The listing builds one solid part. Answer for the finished solid, in the listing's coordinates (mm). Face numbers are marked on the shaded views. A direction names the side the tool comes from. Coordinates: 2 decimals unless noted, no trailing zeros. Loops run counter-clockwise (first coordinate to the right, second up) from the corner with the lowest first, then second, coordinate; pieces in that order, holes last. Notation, with made-up numbers: (74, 51) -> (83, 51) arc R22 cw to (83, 65) -> close; hole circle Ø2 at (-38.75, -17). An arc over 180 degrees is marked (long way). Answer in a Markdown table with one row per item.
```python
from build123d import *

# Parameters (mm, degrees)
SKETCH1_R                                         = 40
SKETCH1_R_2                                       = 26
BOSS_EXTRUDE1_DEPTH                               = 82
BOSS_EXTRUDE2_DEPTH                               = 20
SKETCH4_R                                         = 26
CUT_EXTRUDE1_DEPTH                                = 22
CBORE_FOR_M10_HEX_HEAD_BOLT2_D                    = 13
CBORE_FOR_M10_HEX_HEAD_BOLT2_CBORE_D              = 22
CBORE_FOR_M10_HEX_HEAD_BOLT2_CBORE_DEPTH          = 8
FILLET1_R                                         = 8
CSK_FOR_M10_FLAT_HEAD_MACHINE_SCREW12_D           = 10
CSK_FOR_M10_FLAT_HEAD_MACHINE_SCREW12_DEPTH       = 30
CSK_FOR_M10_FLAT_HEAD_MACHINE_SCREW12_CSINK_D     = 22
CSK_FOR_M10_FLAT_HEAD_MACHINE_SCREW12_CSINK_ANGLE = 50
CSK_FOR_M10_FLAT_HEAD_MACHINE_SCREW12_TIP         = 3.004303095
SKETCH22_R                                        = 30
CUT_EXTRUDE2_DEPTH                                = 6


with BuildPart() as part:
    # Sketch1 → Boss-Extrude1 (new body)
    with BuildSketch(Plane(origin=(0, 0, 0), x_dir=(0, 1, 0), z_dir=(0, 0, 1))):
        with Locations(Location((0, 0, 0), (0, 0, 270))):
            Circle(SKETCH1_R)
        with Locations(Location((0, 0, 0), (0, 0, 270))):
            Circle(SKETCH1_R_2, mode=Mode.SUBTRACT)
    extrude(amount=BOSS_EXTRUDE1_DEPTH)

    # Sketch2 → Boss-Extrude2 (add)
    with BuildSketch(Plane(origin=(0, 0, 0), x_dir=(0, 1, 0), z_dir=(0, 0, 1))):
        with BuildLine():
            Line((-73.617309286, 3.070026527), (-11.117309286, 72.070026527))
            ThreePointArc((-11.117309286, 72.070026527), (0, 77), (11.117309286, 72.070026527))
            Line((11.117309286, 72.070026527), (73.617309286, 3.070026527))
            ThreePointArc((73.617309286, 3.070026527), (76.212228081, -13.080690837), (62.5, -22))
            Line((62.5, -22), (33.406586177, -22))
            ThreePointArc((33.406586177, -22), (0, -40), (-33.406586177, -22))
            Line((-33.406586177, -22), (-62.5, -22))
            ThreePointArc((-62.5, -22), (-76.212228081, -13.080690837), (-73.617309286, 3.070026527))
        make_face()
    extrude(amount=BOSS_EXTRUDE2_DEPTH)

    # Sketch4 → Cut-Extrude1 (cut)
    with BuildSketch(Plane.XY.offset(20)):
        Circle(SKETCH4_R)
    extrude(amount=-CUT_EXTRUDE1_DEPTH, mode=Mode.SUBTRACT)

    # CBORE for M10 Hex Head Bolt2 (through all)
    with Locations(Plane(origin=(-62, 0, 20), x_dir=(1, 0, 0), z_dir=(0, 0, 1))):
        with Locations((0, 0), (69, 62.5), (69, -62.5)):
            CounterBoreHole(CBORE_FOR_M10_HEX_HEAD_BOLT2_D / 2, CBORE_FOR_M10_HEX_HEAD_BOLT2_CBORE_D / 2, CBORE_FOR_M10_HEX_HEAD_BOLT2_CBORE_DEPTH)

    # Fillet1
    fillet1_edges = [part.edges().sort_by_distance(p)[0] for p in [
        (-40, 0, 82),
    ]]
    fillet(fillet1_edges, radius=FILLET1_R)

    # CSK for M10 Flat Head Machine Screw12
    with Locations(Plane.YZ.offset(40)):
        with Locations((0, 50)):
            CounterSinkHole(CSK_FOR_M10_FLAT_HEAD_MACHINE_SCREW12_D / 2, CSK_FOR_M10_FLAT_HEAD_MACHINE_SCREW12_CSINK_D / 2, depth=CSK_FOR_M10_FLAT_HEAD_MACHINE_SCREW12_DEPTH, counter_sink_angle=CSK_FOR_M10_FLAT_HEAD_MACHINE_SCREW12_CSINK_ANGLE)
            with Locations((0, 0, -(CSK_FOR_M10_FLAT_HEAD_MACHINE_SCREW12_DEPTH + CSK_FOR_M10_FLAT_HEAD_MACHINE_SCREW12_TIP / 2))):  # 118° drill point
                Cone(0, CSK_FOR_M10_FLAT_HEAD_MACHINE_SCREW12_D / 2, CSK_FOR_M10_FLAT_HEAD_MACHINE_SCREW12_TIP, mode=Mode.SUBTRACT)

    # Sketch22 → Cut-Extrude2 (cut)
    with BuildSketch(Plane(origin=(0, 0, 0), x_dir=(1, 0, 0), z_dir=(0, 0, -1))):
        with Locations(Location((0, 0, 0), (0, 0, 180))):
            Circle(SKETCH22_R)
    extrude(amount=-CUT_EXTRUDE2_DEPTH, mode=Mode.SUBTRACT)


solid = part.part
```
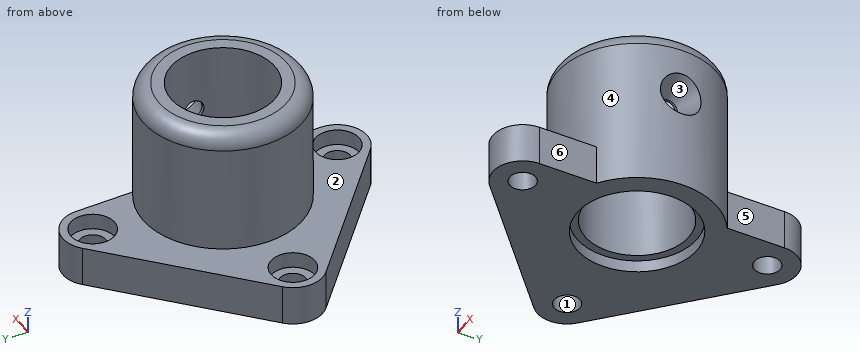
Item 1: Find the intervals of material crossed by probe 1 along X at (y, z) = (2.5, 76.5); probe 2 along Y at (x, z) = (-6, 62); probe 3 along X at (y, z) = (-18, 63), in increasing order.
Findings below:
| item | result |
|---|---|
| probe 1 | x = -39.52 to -25.88, 25.88 to 39.52 |
| probe 2 | y = -39.55 to -25.3, 25.3 to 39.55 |
| probe 3 | x = -35.72 to -18.76, 18.76 to 35.72 |
Item 2: A cutting plane is placed at A-A, the plane y = -59. Determine the outline of the cut face in (x, z).
Findings below:
| item | result |
|---|---|
| outline | (-19.21, 0) -> (1.52, 0) -> (1.52, 12) -> (-3.43, 12) -> (-3.43, 20) -> (-19.21, 20) -> close; (12.48, 0) -> (22, 0) -> (22, 20) -> (17.43, 20) -> (17.43, 12) -> (12.48, 12) -> close |
Item 3: A cutting plane is placed at D-D, the plane x = 7. Count the separate pieces of the cut face and the enclosed holes in it, plus the area to 3 significant figures.
Findings below:
| item | result |
|---|---|
| separate pieces | 4 |
| enclosed holes | 0 |
| area | 3,140 mm2 |
Item 4: A cutting plane is placed at B-B, the plane x = -57.5. Determine the outline of the cut face in (y, z).
Findings below:
| item | result |
|---|---|
| outline | (-24.31, 0) -> (-4.69, 0) -> (-4.69, 12) -> (-10.04, 12) -> (-10.04, 20) -> (-24.31, 20) -> close; (4.69, 0) -> (24.31, 0) -> (24.31, 20) -> (10.04, 20) -> (10.04, 12) -> (4.69, 12) -> close |
Item 5: A tool of negligible diameter and unlimited length cuts with its end or side. For the marked faces 4, 5 and 6, from which of +Z, -Z, +X, -X, +Y, -Y can it reach the whole face along a straight path? Write none if from no direction.
Findings below:
| item | result |
|---|---|
| face 4 | +Z |
| face 5 | +Z, -Z, +X, +Y |
| face 6 | +Z, -Z, +X, -Y |
Item 6: Determine the mould class of the marked faces 1, 2 and 3 for opening direction Z: +Z half, -Z half, draft (parallel to the pull), parting line (faces both ways), or undercut.
Findings below:
| item | result |
|---|---|
| face 1 | draft |
| face 2 | +Z half |
| face 3 | undercut |
Item 7: Flat-ended cylindrical pins translate along their axes: pin 1 Ø17.5 at (x, y) = (4, -67.5) entering from +Z; pin 2 Ø11.5 at (x, y) = (7, 62.5) entering from -Z; pin 3 Ø5 at (x, z) = (-13.5, 62.5) entering from -Y; pin 4 Ø15 at (x, y) = (-62, 0) entering from +Z. Find the tip coordinate at first contact, or state that the pin passes through.
Findings below:
| item | result |
|---|---|
| pin 1 | stops at z = 20 |
| pin 2 | passes through |
| pin 3 | stops at y = -38.46 |
| pin 4 | stops at z = 12 |
Item 8: A cutting plane is placed at C-C, the plane z = 33.5. Determine the outline of the cut face in (x, y).
Findings below:
| item | result |
|---|---|
| outline | circle Ø80 at (0, 0); hole circle Ø52 at (0, 0) |
